```python
from build123d import *

# Parameters (mm, degrees)
BOSS_EXTRUDE1_DEPTH      = 63.5
BOSS_EXTRUDE1_DEPTH_BACK = 63.5
CUT_EXTRUDE1_REACH       = 573.246
SKETCH4_W                = 12.7
SKETCH4_H                = 12.7
BOSS_EXTRUDE3_DEPTH      = 4.7625
CUT_EXTRUDE2_DEPTH       = 467.787091958
CUT_EXTRUDE2_DEPTH_BACK  = 467.787091958
SKETCH11_RX              = 177.8
SKETCH11_RY              = 25.4


with BuildPart() as part:
    # Sketch2 → Boss-Extrude1 (new, two sides: drawn at the far end of the back side and taken through both)
    with BuildSketch(Plane(origin=(0, 0, 0), x_dir=(0, 0, -1), z_dir=(1, 0, 0)).offset(-BOSS_EXTRUDE1_DEPTH_BACK)):
        with BuildLine():
            Line((0, -4.7625), (-398.4625, -4.7625))
            Line((-398.4625, -4.7625), (-398.4625, 233.3625))
            Line((-398.4625, 233.3625), (0, 233.3625))
            ThreePointArc((0, 233.3625), (119.0625, 114.3), (0, -4.7625))
        make_face()
        with BuildLine():
            Line((0, 0), (-393.7, 0))
            Line((-393.7, 0), (-393.7, 228.6))
            Line((-393.7, 228.6), (0, 228.6))
            ThreePointArc((0, 228.6), (114.3, 114.3), (0, 0))
        make_face(mode=Mode.SUBTRACT)
    extrude(amount=BOSS_EXTRUDE1_DEPTH + BOSS_EXTRUDE1_DEPTH_BACK)

    # Sketch4 → Cut-Extrude1 (cut, up to next)
    with BuildSketch(Plane.XY.offset(398.4625), mode=Mode.PRIVATE) as cut_extrude1_sk1:
        with Locations((0, 19.05)):
            Rectangle(SKETCH4_W, SKETCH4_H)
    cut_extrude1_tool1 = extrude(cut_extrude1_sk1.sketch, amount=-CUT_EXTRUDE1_REACH, mode=Mode.PRIVATE) & part.part
    add(cut_extrude1_tool1.solids().sort_by_distance((0, 19.05, 398.4625))[0], mode=Mode.SUBTRACT)

    # Sketch9 → Boss-Extrude3 (add)
    with BuildSketch(Plane(origin=(63.5, 0, 0), x_dir=(0, 0, -1), z_dir=(1, 0, 0))):
        with BuildLine():
            Line((-398.4625, 233.3625), (0, 233.3625))
            ThreePointArc((0, 233.3625), (119.0625, 114.3), (0, -4.7625))
            Line((0, -4.7625), (-398.4625, -4.7625))
            Line((-398.4625, -4.7625), (-398.4625, 233.3625))
        make_face()
    boss_extrude3 = extrude(amount=BOSS_EXTRUDE3_DEPTH)

    # Mirror1: Boss-Extrude3 across plane
    add(boss_extrude3.mirror(Plane(origin=(0, 0, 0), x_dir=(0, 0, 1), z_dir=(1, 0, 0))))

    # Sketch11 → Cut-Extrude2 (cut, two sides: drawn at the far end of the back side and taken through both)
    with BuildSketch(Plane(origin=(0, 0, 0), x_dir=(0, 0, -1), z_dir=(1, 0, 0)).offset(-CUT_EXTRUDE2_DEPTH_BACK)):
        with Locations(Location((-220.6625, 233.3625), (0, 0, -180))):
            Ellipse(SKETCH11_RX, SKETCH11_RY)
    extrude(amount=CUT_EXTRUDE2_DEPTH + CUT_EXTRUDE2_DEPTH_BACK, mode=Mode.SUBTRACT)


solid = part.part
```
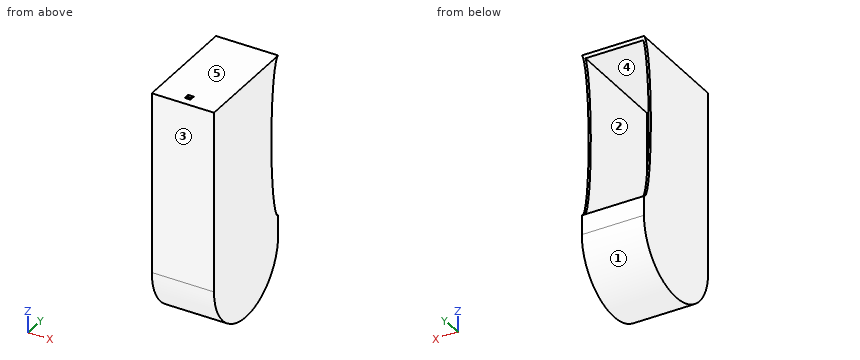
The listing builds one solid part. Answer for the finished solid, in the listing's coordinates (mm). Face numbers are marked on the shaded views. A direction names the side the tool comes from. Give positions to 0.01 mm unless a question says otherwise; leave off trailing zeros. Order: outer loops, then holes, each group sorted by start corner. A loop starts at its lowest first (then second) coordinate and runs counter-clockwise, first axis right, second up. Notation, with made-up numbers: (45.5, 13) -> (96.5, 13) arc R12 cw to (96.5, 34) -> close; hole circle Ø6 at (-2, 38). An arc over 180 degrees is marked (long way). One line per item, written item: value.
1) A tool of negligible diameter and unlimited length cuts with its end or side. For the marked faces 4 and 5, from which of +Z, -Z, +X, -X, +Y, -Y can it reach the whole face along a straight path? Write none if from no direction.
Reported:
face 4: +Y
face 5: +Z, +X, -X, +Y, -Y
2) Find the intervals of material crossed by line 1 (Y direction, x = -33.5, z = 3); line 2 (Z direction, x = -3, y = 113); line 3 (X direction, y = 86, z = 4), in increasing order.
Reported:
line 1: y = -4.76 to 0, 228.6 to 233.36
line 2: z = -119.06 to -114.29, 393.7 to 398.46
line 3: x = -68.26 to -63.5, 63.5 to 68.26
3) Determine the mould class of the marked faces 1, 2 and 3 for opening direction Z: pulls with the +Z half, pulls with the -Z half, needs draft (parallel to the pull), parting line crosses it, or undercut.
Reported:
face 1: pulls with the -Z half
face 2: undercut
face 3: needs draft
4) Flat-ended cylindrical pins translate along their axes: P1, Ø2.5, axis at x = 2, z = 395.5, coming from the +Y side; P2, Ø10, axis at x = -45.5, y = 138.5, coming from the -Z side; P3, Ø4, axis at x = -37.5, y = 27.5, coming from the -Z side. Find the tip coordinate at first contact, or state that the pin passes through.
Reported:
P1: stops at y = 229.85
P2: stops at z = -117.5
P3: stops at z = -83.58
5) Find section A-A, the plane z = 34.5. Determine the outline of the cut face in (x, y).
Reported:
outline: (-68.26, -4.76) -> (68.26, -4.76) -> (68.26, 233.36) -> (-68.26, 233.36) -> close; hole (-63.5, 0) -> (63.5, 0) -> (63.5, 228.6) -> (-63.5, 228.6) -> close
6) Find section B-B, the plane y = 51. Determine the outline of the cut face in (x, z).
Reported:
outline: (-68.26, -100.84) -> (68.26, -100.84) -> (68.26, 398.46) -> (-68.26, 398.46) -> close; hole (-63.5, -95.17) -> (63.5, -95.17) -> (63.5, 393.7) -> (-63.5, 393.7) -> close
